Could you check a few things on this drawing? It's one solid part, dimensions in mm from its lowest x, y, z. Coordinates: 2 decimals unless noted, no trailing zeros. Order: outer loops, then holes, each group sorted by start corner. A loop starts at its lowest first (then second) coordinate and runs counter-clockwise, first axis right, second up.
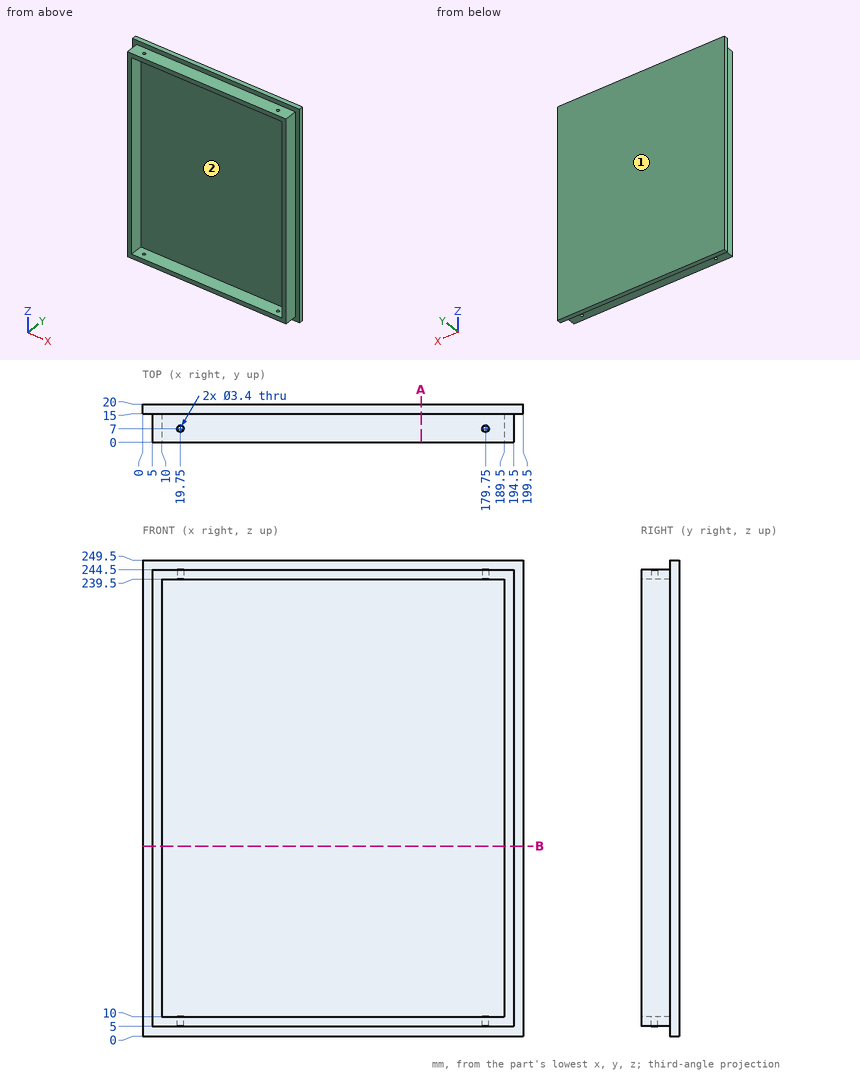
Item 1: I need wall thicknesses on line 1 (X direction, y = 7, z = 8.8); line 2 (X direction, y = 1.5, z = 28.5); line 3 (Z direction, x = 163, y = 14.75). Which ranges of each line are inside material? Lowest first, please.
Item 2: Suppose I cut it at A-A (x = 146). List the corners of the cut face in (y, z) for me.
Item 3: Suppose I cut it at B-B (z = 99.5). List the corners of the cut face in (x, y) for me, and give its area (3 significant figures).
Item 4: Thinking about a two-plate mould opening in X: for the marked faces 1 and 2, which applies, +X half, -X half, draft (parallel to the pull), parting line (faces both ways), or undercut?
Item 5: For pin 1 Ø12 at (y, z) = (8, 101) entering from -X; pin 2 Ø8 at (y, z) = (12.5, 44) entering from -X; pin 3 Ø2 at (y, z) = (12, 223) entering from +X; pin 4 Ø10 at (x, z) = (56.5, 77) entering from -Y, each with a flat end and sliding along its axis, tell me the tip position at first contact or that it passes through.
Geometry results:
1. line 1: x = 5 to 18.05, 21.45 to 178.05, 181.45 to 194.5
1. line 2: x = 5 to 10, 189.5 to 194.5
1. line 3: z = 5 to 10, 239.5 to 244.5
2. outline: (0, 5) - (15, 5) - (15, 0) - (20, 0) - (20, 249.5) - (15, 249.5) - (15, 244.5) - (0, 244.5) - (0, 239.5) - (15, 239.5) - (15, 10) - (0, 10) - close
3. outline: (0, 15) - (5, 15) - (5, 0) - (10, 0) - (10, 15) - (189.5, 15) - (189.5, 0) - (194.5, 0) - (194.5, 15) - (199.5, 15) - (199.5, 20) - (0, 20) - close
3. area: 1,150 mm2
4. face 1: draft
4. face 2: undercut
5. pin 1: stops at x = 5
5. pin 2: stops at x = 0
5. pin 3: stops at x = 194.5
5. pin 4: stops at y = 15
